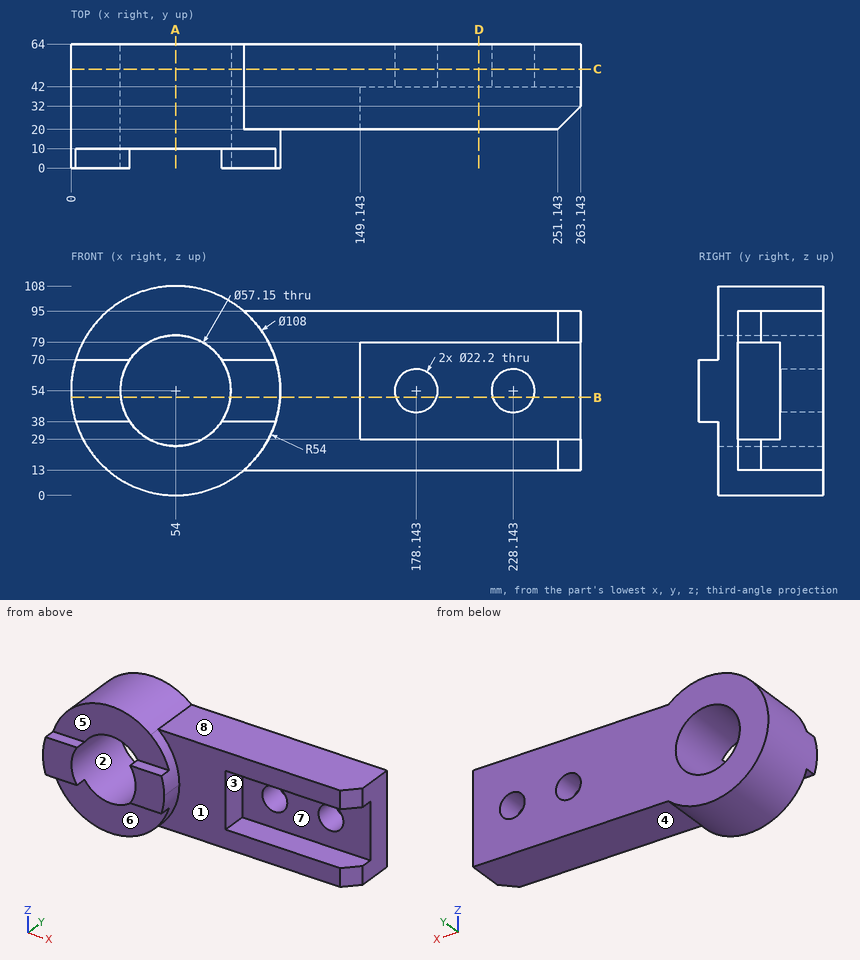
Can you work these out from the drawing? Everything is in mm from the part's minimum corner. A direction names the side the tool comes from. Give positions to 0.01 mm unless a question says otherwise; leave off trailing zeros. Loops run counter-clockwise (first coordinate to the right, second up) from the corner with the lowest first, then second, coordinate; pieces in that order, holes last. Notation, with made-up numbers: (6, 37) -> (12, 37) arc R27 cw to (12, 68) -> close; hole circle Ø3 at (15, -25.5). An arc over 180 degrees is marked (long way). Return JSON: item names as keys, results as strings.
Item 1: If we section it at B-B on z = 50.5: List the corners of the cut face in (x, y) for me.
Geometry results:
{"outline": "(0.11, 0) -> (25.64, 0) -> (25.64, 64) -> (0.11, 64) -> close; (82.36, 0) -> (107.89, 0) -> (107.89, 20) -> (149.14, 20) -> (149.14, 42) -> (167.61, 42) -> (167.61, 64) -> (82.36, 64) -> close; (188.68, 42) -> (217.61, 42) -> (217.61, 64) -> (188.68, 64) -> close; (238.68, 42) -> (263.14, 42) -> (263.14, 64) -> (238.68, 64) -> close"}
Item 2: If we section it at A-A on x = 54: List the corners of the cut face in (y, z) for me (1 decimal), plus the area to 3 significant figures.
Geometry results:
{"outline": "(10, 0) -> (64, 0) -> (64, 25.4) -> (10, 25.4) -> close; (10, 82.6) -> (64, 82.6) -> (64, 108) -> (10, 108) -> close", "area": "2,750 mm²"}
Item 3: If we section it at D-D on x = 210.5: List the corners of the cut face in (y, z) for me.
Geometry results:
{"outline": "(20, 13) -> (64, 13) -> (64, 95) -> (20, 95) -> (20, 79) -> (42, 79) -> (42, 29) -> (20, 29) -> close"}
Item 4: I'm going to push flat-ended pins straight in: pin 1 (6 mm diameter, centred on y = 16, z = 44, fed in from +X) (1 decimal); pin 2 (22 mm diameter, centred on x = 169.5, y = 46.5, fed in from -Z); pin 3 (6 mm diameter, centred on x = 149, z = 71.5, fed in from -Y). Where does each tip first touch, or does it pass through?
Geometry results:
{"pin 1": "stops at x = 107.5", "pin 2": "stops at z = 13", "pin 3": "stops at y = 20"}
Item 5: If we section it at C-C on y = 51: Count the separate pieces of the cut face and the enclosed holes in it, plus the area to 3 significant figures.
Geometry results:
{"separate pieces": "1", "enclosed holes": "3", "area": "19,000 mm²"}
Item 6: I need wall thicknesses on L1, parallel to Z at x = 54, y = 35 (1 decimal); L2, parallel to Z at x = 217, y = 34.5; L3, parallel to Y at x = 245, z = 59. Which ranges of each line are inside material? Lowest first, please. Write a range as from..to.
Geometry results:
{"L1": "z = 0..25.4, 82.6..108", "L2": "z = 13..29, 79..95", "L3": "y = 42..64"}
Item 7: We'd pull the mould along X, two halves only. Please class the marked faces 1, 2 and 3: +X half, -X half, draft (parallel to the pull), parting line (faces both ways), or undercut.
Geometry results:
{"face 1": "draft", "face 2": "undercut", "face 3": "+X half"}
Item 8: Which directions (+Z, -Z, +X, -X, +Y, -Y) give clear straight access to the entire face, cutting with the end or side of a thin tool? Please do the marked faces 4, 5, 6, 7 and 8.
Geometry results:
{"face 4": "-Z, +X, +Y, -Y", "face 5": "+Z, +X, -X, -Y", "face 6": "-Z, +X, -X, -Y", "face 7": "+X, -Y", "face 8": "+Z, +X, +Y, -Y"}
